```python
from build123d import *

# Parameters (mm, degrees)
CHAMFER1_SIZE  = 1
CHAMFER1_SIZE2 = 1.161440479
FILLET1_R      = 0.5


with BuildPart() as part:
    # Sketch1 → Revolve1 (revolve)
    with BuildSketch(Plane(origin=(0, 0, 0), x_dir=(0, 0, -1), z_dir=(1, 0, 0)), mode=Mode.PRIVATE) as revolve1_sk:
        Polygon((0, -95), (40, -95), (52.5, 0), (55.525858089, 0), (42.631121247, -98), (0, -98), align=None)
    revolve(revolve1_sk.sketch.rotate(Axis((0, 0, 0), (0, -1, 0)), 180), axis=Axis((0, 0, 0), (0, -1, 0)))

    # Chamfer1
    chamfer1_edges = [part.edges().sort_by_distance(p)[0] for p in [
        (0, -98, -42.631121247),
    ]]
    chamfer1_side = [part.faces().sort_by_distance(p)[0] for p in [
        (0, -98, 0),
    ]]
    chamfer(chamfer1_edges, length=CHAMFER1_SIZE, length2=CHAMFER1_SIZE2, reference=chamfer1_side[0])

    # Fillet1
    fillet1_edges = [part.edges().sort_by_distance(p)[0] for p in [
        (0, 0, -52.5),
        (0, 0, -55.525858089),
    ]]
    fillet(fillet1_edges, radius=FILLET1_R)


solid = part.part
```
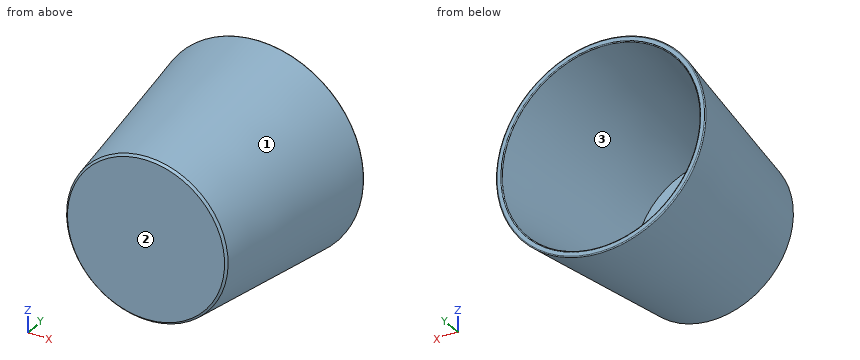
Input: part model. Units: mm. Frame: model coordinates. Face numbers are marked on the shaded views. Coordinates: 2 decimals unless noted, no trailing zeros. Loops run counter-clockwise (first coordinate to the right, second up) from the corner with the lowest first, then second, coordinate; pieces in that order, holes last. Notation, with made-up numbers: M -19.5,-24 L 0.5,-24 A15 cw 0.5,-5 Z; hole C -30.75,-18.5 d10. An arc over 180 degrees is marked long. One line per item, written item: value.
(1) Pull-direction query (Z, two-part tool) for the marked faces 1, 2 and 3; classes: +Z half, -Z half, draft (parallel to the pull), parting line (faces both ways), or undercut.
Filled in:
face 1: parting line
face 2: draft
face 3: undercut
(2) Line query: line 1 along Y through (x, z) = (27, 26); line 2 along X through (y, z) = (-58, -36.5); line 3 along X through (y, z) = (-70, 19.5). Output: solid intervals per line, ascending. Write a range as from..to.
Filled in:
line 1: -98..-95
line 2: -31.01..-26.09, 26.09..31.01
line 3: -42.01..-38.65, 38.65..42.01
(3) Section C-C (y = -66). Output: boundary loops of the cut face in (x, z), and give its area (3 significant figures).
Filled in:
outline: C 0,0 d93.68; hole C 0,0 d87.63
area: 862 mm^2
(4) Section B-B (x = 0). Output: boundary loops of the cut face in (y, z), and give its area (3 significant figures).
Filled in:
outline: M -98,-41.63 L -96.85,-42.78 L -0.57,-55.45 A0.5 ccw 0,-54.96 L 0,-52.94 A0.5 ccw -0.43,-52.44 L -95,-40 L -95,40 L -0.43,52.44 A0.5 ccw 0,52.94 L 0,54.96 A0.5 ccw -0.57,55.45 L -96.85,42.78 L -98,41.63 Z
area: 831 mm^2
(5) Section D-D (y = -28.5). Output: boundary loops of the cut face in (x, z), and give its area (3 significant figures).
Filled in:
outline: C 0,0 d103.55; hole C 0,0 d97.5
area: 956 mm^2
(6) Section A-A (z = 0). Output: boundary loops of the cut face in (x, y).
Filled in:
outline: M -55.45,-0.57 L -42.78,-96.85 L -41.63,-98 L 41.63,-98 L 42.78,-96.85 L 55.45,-0.57 A0.5 ccw 54.96,0 L 52.94,0 A0.5 ccw 52.44,-0.43 L 40,-95 L -40,-95 L -52.44,-0.43 A0.5 ccw -52.94,0 L -54.96,0 A0.5 ccw Z
(7) Pin query (flat end, axial travel): pin 1 (1.5 mm diameter, centred on y = -60.5, z = -2.5, fed in from +X); pin 2 (3 mm diameter, centred on x = 33.5, y = -72, fed in from -Z); pin 3 (8 mm diameter, centred on y = -71, z = 30, fed in from -X). Return the tip coordinate at first contact, or that it passes through.
Filled in:
pin 1: x = 47.61
pin 2: z = -33.14
pin 3: x = -38.24
